Work out the finished part from the listing and answer in its coordinate system (mm). Face numbers are marked on the shaded views. A direction names the side the tool comes from. Give positions to 0.01 mm unless a question says otherwise; leave off trailing zeros. Loops run counter-clockwise (first coordinate to the right, second up) from the corner with the lowest first, then second, coordinate; pieces in that order, holes last. Notation, with made-up numbers: (24.25, -29) -> (59.25, -29) arc R32 ccw to (59.25, 1) -> close; hole circle Ø3 at (75, 69.5). An arc over 180 degrees is marked (long way). Answer as CSV lines item,"result". Start each with the question number.
1. Flat-ended cylindrical pins translate along their axes: pin 1 Ø12 at (x, y) = (0, 0) entering from +Z; pin 2 Ø5 at (x, y) = (-13, 11.5) entering from +Z; pin 3 Ø15 at (x, z) = (-6.5, 121.5) entering from +Y; pin 4 Ø1.6 at (x, z) = (-10.5, 2) entering from +Y. Find the tip coordinate at first contact, or state that the pin passes through.
2. Find the intervals of material crossed by line 1 along X through (y, z) = (-11, 115); line 2 along X through (y, z) = (11.7, 2.5); line 3 along X through (y, z) = (-10, 32), in increasing order.
3. Find section A-A, the plane z = 86.5. Give the vertices of the cut face in (x, y), and give its area (3 significant figures).
4. A tool of negligible diameter and unlimited length cuts with its end or side. For the marked faces 1 and 2, from which of +Z, -Z, +X, -X, +Y, -Y can it reach the whole face along a straight path? Write none if from no direction.
5. Find section B-B, the plane z = 38.5. Count the separate pieces of the cut face and the enclosed holes in it, and give its area (3 significant figures).
from build123d import *

# Parameters (mm, degrees)
SKETCH_1_W          = 50
SKETCH_1_H          = 29
SKETCH_1_R          = 1.5
SKETCH_1_R_2        = 7.5
EXTRUDE_1_DEPTH     = 5
SKETCH_22_W         = 50
SKETCH_22_H         = 10
EXTRUDE_2_DEPTH     = 30
EXTRUDE_3_DEPTH     = 10
SKETCH_25_R         = 5
SKETCH_25_R_2       = 1.5
CUT_EXTRUDE_1_DEPTH = 144.478221472
SKETCH_26_R         = 0.75
CUT_EXTRUDE_2_DEPTH = 5


with BuildPart() as part:
    # 草圖1 → 填料-伸長1 (new body)
    with BuildSketch(Plane.XY):
        Rectangle(SKETCH_1_W, SKETCH_1_H)
        with Locations((0, 10)):
            Circle(SKETCH_1_R, mode=Mode.SUBTRACT)
        with Locations((-8.660254038, -5)):
            Circle(SKETCH_1_R, mode=Mode.SUBTRACT)
        with Locations((8.660254038, -5)):
            Circle(SKETCH_1_R, mode=Mode.SUBTRACT)
        Circle(SKETCH_1_R_2, mode=Mode.SUBTRACT)
    extrude(amount=EXTRUDE_1_DEPTH)

    # 疊層拉伸2: read off the stored shape, not the designer's step
    # 疊層拉伸2: loft between two sections, ruled curve by curve
    loft_2_from = [
        Edge.make_bspline([(-13, 10, 55), (-13, 6.666666667, 55), (-13, 3.333333333, 55), (-13, -3.333333333, 55), (-13, -6.666666667, 55), (-13, -10, 55)], [0, 0, 0, 0, 0.5, 0.5, 1, 1, 1, 1], 3),
        Edge.make_bspline([(-13, -10, 55), (-15, -10, 55), (-17, -10, 55), (-21, -10, 55), (-23, -10, 55), (-25, -10, 55)], [0, 0, 0, 0, 0.5, 0.5, 1, 1, 1, 1], 3),
        Edge.make_bspline([(-25, 10, 55), (-23, 10, 55), (-21, 10, 55), (-17, 10, 55), (-15, 10, 55), (-13, 10, 55)], [0, 0, 0, 0, 0.5, 0.5, 1, 1, 1, 1], 3),
        Edge.make_bspline([(-25, -10, 55), (-25, -6.666666667, 55), (-25, -3.333333333, 55), (-25, 3.333333333, 55), (-25, 6.666666667, 55), (-25, 10, 55)], [0, 0, 0, 0, 0.5, 0.5, 1, 1, 1, 1], 3),
    ]
    loft_2_to = [
        Edge.make_bspline([(-25, 14.5, 5), (-23, 14.5, 5), (-21, 14.5, 5), (-17, 14.5, 5), (-15, 14.5, 5), (-13, 14.5, 5)], [0, 0, 0, 0, 0.5, 0.5, 1, 1, 1, 1], 3),
        Edge.make_bspline([(-13, 14.5, 5), (-13, 9.666666667, 5), (-13, 4.833333333, 5), (-13, -4.833333333, 5), (-13, -9.666666667, 5), (-13, -14.5, 5)], [0, 0, 0, 0, 0.5, 0.5, 1, 1, 1, 1], 3),
        Edge.make_bspline([(-25, -14.5, 5), (-25, -9.666666667, 5), (-25, -4.833333333, 5), (-25, 4.833333333, 5), (-25, 9.666666667, 5), (-25, 14.5, 5)], [0, 0, 0, 0, 0.5, 0.5, 1, 1, 1, 1], 3),
        Edge.make_bspline([(-13, -14.5, 5), (-15, -14.5, 5), (-17, -14.5, 5), (-21, -14.5, 5), (-23, -14.5, 5), (-25, -14.5, 5)], [0, 0, 0, 0, 0.5, 0.5, 1, 1, 1, 1], 3),
    ]
    loft_2 = Solid(Shell([*[Face.make_surface_from_curves(loft_2_from[k], loft_2_to[k]) for k in range(4)], Face(Wire(loft_2_from)), Face(Wire(loft_2_to))]))
    add(loft_2)

    # 疊層拉伸7: read off the stored shape, not the designer's step
    # 疊層拉伸7: loft between two sections, ruled curve by curve
    loft_7_from = [
        Edge.make_bspline([(-0.1, -8.5, 5), (-2.25, -8.5, 5), (-4.4, -8.5, 5), (-8.7, -8.5, 5), (-10.85, -8.5, 5), (-13, -8.5, 5)], [0, 0, 0, 0, 0.5, 0.5, 1, 1, 1, 1], 3),
        Edge.make_bspline([(-13, -8.5, 5), (-13, -9.5, 5), (-13, -10.5, 5), (-13, -12.5, 5), (-13, -13.5, 5), (-13, -14.5, 5)], [0, 0, 0, 0, 0.5, 0.5, 1, 1, 1, 1], 3),
        Edge.make_bspline([(-0.1, -14.5, 5), (-0.1, -13.5, 5), (-0.1, -12.5, 5), (-0.1, -10.5, 5), (-0.1, -9.5, 5), (-0.1, -8.5, 5)], [0, 0, 0, 0, 0.5, 0.5, 1, 1, 1, 1], 3),
        Edge.make_bspline([(-13, -14.5, 5), (-10.85, -14.5, 5), (-8.7, -14.5, 5), (-4.4, -14.5, 5), (-2.25, -14.5, 5), (-0.1, -14.5, 5)], [0, 0, 0, 0, 0.5, 0.5, 1, 1, 1, 1], 3),
    ]
    loft_7_to = [
        Edge.make_bspline([(-10.1, -8.5, 55), (-10.1, -9.5, 55), (-10.1, -10.5, 55), (-10.1, -12.5, 55), (-10.1, -13.5, 55), (-10.1, -14.5, 55)], [0, 0, 0, 0, 0.5, 0.5, 1, 1, 1, 1], 3),
        Edge.make_bspline([(-10.1, -14.5, 55), (-8.433333333, -14.5, 55), (-6.766666667, -14.5, 55), (-3.433333333, -14.5, 55), (-1.766666667, -14.5, 55), (-0.1, -14.5, 55)], [0, 0, 0, 0, 0.5, 0.5, 1, 1, 1, 1], 3),
        Edge.make_bspline([(-0.1, -8.5, 55), (-1.766666667, -8.5, 55), (-3.433333333, -8.5, 55), (-6.766666667, -8.5, 55), (-8.433333333, -8.5, 55), (-10.1, -8.5, 55)], [0, 0, 0, 0, 0.5, 0.5, 1, 1, 1, 1], 3),
        Edge.make_bspline([(-0.1, -14.5, 55), (-0.1, -13.5, 55), (-0.1, -12.5, 55), (-0.1, -10.5, 55), (-0.1, -9.5, 55), (-0.1, -8.5, 55)], [0, 0, 0, 0, 0.5, 0.5, 1, 1, 1, 1], 3),
    ]
    loft_7 = Solid(Shell([*[Face.make_surface_from_curves(loft_7_from[k], loft_7_to[k]) for k in range(4)], Face(Wire(loft_7_from)), Face(Wire(loft_7_to))]))
    add(loft_7)

    # 草圖17 → section 1 of loft_13
    with BuildSketch(Plane.XY.offset(85), mode=Mode.PRIVATE) as loft_13_s1:
        with BuildLine():
            Line((-25, -14.5), (-13, -14.5))
            Line((-13, -14.5), (-13, -4.5))
            Line((-13, -4.5), (-25, -4.5))
            Line((-25, -4.5), (-25, -14.5))
        make_face()
    # loft from a face of the part (loft_13)
    loft([part.faces().sort_by_distance((-19, 0, 55))[0], loft_13_s1.sketch])

    # 草圖19 → section 0 of loft_14
    with BuildSketch(Plane.XY.offset(85), mode=Mode.PRIVATE) as loft_14_s0:
        with BuildLine():
            Line((-12.5, -14.5), (-0.5, -14.5))
            Line((-0.5, -14.5), (-0.5, -4.5))
            Line((-0.5, -4.5), (-12.5, -4.5))
            Line((-12.5, -4.5), (-12.5, -14.5))
        make_face()
    # loft up to a face of the part (loft_14)
    loft([loft_14_s0.sketch, part.faces().sort_by_distance((-5.1, -11.5, 55))[0]])

    # 鏡射5: 疊層拉伸2, 疊層拉伸7 across plane
    add(loft_2.mirror(Plane.ZY))
    add(loft_7.mirror(Plane.ZY))

    # 草圖20 → section 0 of loft_15
    with BuildSketch(Plane.XY.offset(85), mode=Mode.PRIVATE) as loft_15_s0:
        with BuildLine():
            Line((25, -4.5), (13, -4.5))
            Line((13, -4.5), (13, -14.5))
            Line((13, -14.5), (25, -14.5))
            Line((25, -14.5), (25, -4.5))
        make_face()
    # loft up to a face of the part (loft_15)
    loft([loft_15_s0.sketch, part.faces().sort_by_distance((19, 0, 55))[0]])

    # 草圖21 → section 1 of loft_16
    with BuildSketch(Plane.XY.offset(85), mode=Mode.PRIVATE) as loft_16_s1:
        with BuildLine():
            Line((0.1, -14.5), (12.9, -14.5))
            Line((12.9, -14.5), (12.9, -4.5))
            Line((12.9, -4.5), (0.1, -4.5))
            Line((0.1, -4.5), (0.1, -14.5))
        make_face()
    # loft from a face of the part (loft_16)
    loft([part.faces().sort_by_distance((5.1, -11.5, 55))[0], loft_16_s1.sketch])

    # 草圖22 → 填料-伸長2 (add)
    with BuildSketch(Plane.XY.offset(85)):
        with Locations((0, -9.5)):
            Rectangle(SKETCH_22_W, SKETCH_22_H)
    extrude(amount=EXTRUDE_2_DEPTH)

    # 草圖23 → 填料-伸長3 (add)
    with BuildSketch(Plane(origin=(0, -4.5, 0), x_dir=(1, 0, 0), z_dir=(0, 1, 0))):
        with BuildLine():
            Line((-25, -115), (25, -115))
            ThreePointArc((25, -115), (0, -140), (-25, -115))
        make_face()
    extrude(amount=-EXTRUDE_3_DEPTH)

    # 草圖25 → 除料-伸長1 (cut, through all)
    with BuildSketch(Plane(origin=(0, -4.5, 0), x_dir=(1, 0, 0), z_dir=(0, 1, 0))):
        with Locations(Location((0, -115, 0), (0, 0, 270))):
            Circle(SKETCH_25_R)
        with Locations(Location((9.5, -115, 0), (0, 0, 270))):
            Circle(SKETCH_25_R_2)
        with Locations(Location((-9.5, -115, 0), (0, 0, 270))):
            Circle(SKETCH_25_R_2)
    extrude(amount=-CUT_EXTRUDE_1_DEPTH, mode=Mode.SUBTRACT)

    # 草圖26 → 除料-伸長2 (cut)
    with BuildSketch(Plane(origin=(0, 14.5, 0), x_dir=(1, 0, 0), z_dir=(0, 1, 0))):
        with Locations(Location((-10, -2.5, 0), (0, 0, 270))):
            Circle(SKETCH_26_R)
        with Locations(Location((10, -2.5, 0), (0, 0, 270))):
            Circle(SKETCH_26_R)
    extrude(amount=-CUT_EXTRUDE_2_DEPTH, mode=Mode.SUBTRACT)


solid = part.part
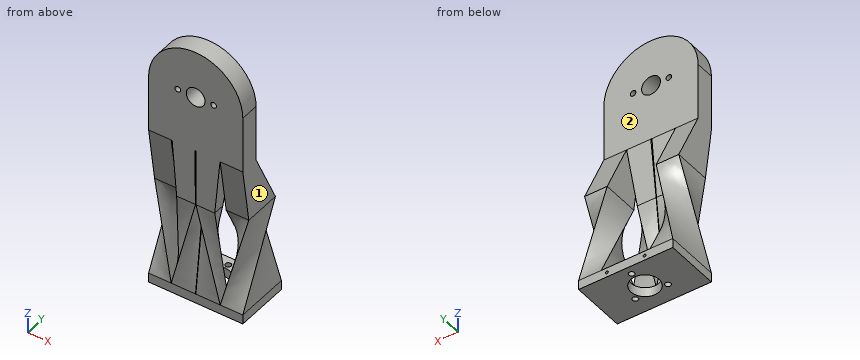
Resolved:
1,pin 1,"stops at z = 140"
1,pin 2,"stops at z = 57.07"
1,pin 3,"stops at y = -4.5"
1,pin 4,"stops at y = 14.5"
2,line 1,"x = -25 to -11, -8 to -5, 5 to 8, 11 to 25"
2,line 2,"x = -25 to -10.75, -9.25 to 9.25, 10.75 to 25"
2,line 3,"x = -20.54 to -18.47, -8.25 to -2.57, 2.57 to 8.25, 18.47 to 20.54"
3,outline,"(-25, -14.5) -> (25, -14.5) -> (25, -4.5) -> (-25, -4.5) -> close"
3,area,"500 mm^2"
4,face 1,"+Z, -Z, +X, +Y, -Y"
4,face 2,"+Z, +X, -X, +Y"
5,separate pieces,"4"
5,enclosed holes,"0"
5,area,"362 mm^2"
